CAD build for the part. Positions are in the model's coordinates, mm. A direction names the side the tool comes from. Coordinates: 2 decimals unless noted, no trailing zeros. Loops run counter-clockwise (first coordinate to the right, second up) from the corner with the lowest first, then second, coordinate; pieces in that order, holes last. Notation, with made-up numbers: (56.25, -17) -> (72.25, -17) arc R26 ccw to (72.25, 8) -> close; hole circle Ø4 at (29, 51.5). An arc over 180 degrees is marked (long way). Write each question's results on one line, items separated by ' | '.
```python
from build123d import *

# Parameters (mm, degrees)
F0_R     = 2.75
F0_R_2   = 1.65
F0_W     = 33
F0_H     = 15.5
F0_R_3   = 2.5
F1_DEPTH = 6
F2_R     = 5
F3_DEPTH = 2
F4_DEPTH = 25


with BuildPart() as f1:
    # F0 (on Top) → F1 (new body, symmetric)
    with BuildSketch(Plane.XY):
        Polygon((4, 14.5), (-4, 14.5), (-4, 10.123076), (-4, 5.690599), (0, 3.381198), (4, 5.690599), (4, 10.309401), align=None)
        with Locations((0, 8)):
            Circle(F0_R, mode=Mode.SUBTRACT)
        Polygon((-4, 14.5), (-16.5, 14.5), (-16.5, 1), (16.5, 1), (16.5, 14.5), (4, 14.5), (4, 10.309401), (4, 5.690599), (0, 3.381198), (-4, 5.690599), (-4, 10.123076), align=None)
        with Locations((-10.15, 8)):
            Circle(F0_R_2, mode=Mode.SUBTRACT)
        with Locations((10.15, 8)):
            Circle(F0_R_2, mode=Mode.SUBTRACT)
        with Locations((0, -6.75)):
            Rectangle(F0_W, F0_H)
        with Locations((-10.379309, -9.5)):
            Circle(F0_R_3, mode=Mode.SUBTRACT)
        with Locations((9.157613, -9.5)):
            Circle(F0_R_3, mode=Mode.SUBTRACT)
    extrude(amount=F1_DEPTH, both=True)

    # F2
    f2_edges = [f1.edges().sort_by_distance(p)[0] for p in [
        (16.5, 14.5, 0),
        (-16.5, 14.5, 0),
    ]]
    fillet(f2_edges, radius=F2_R)

    # F0 (on Top) → F3 (cut, symmetric)
    with BuildSketch(Plane.XY):
        Polygon((4, 14.5), (-4, 14.5), (-4, 10.123076), (-4, 5.690599), (0, 3.381198), (4, 5.690599), (4, 10.309401), align=None)
        with Locations((0, 8)):
            Circle(F0_R, mode=Mode.SUBTRACT)
    extrude(amount=F3_DEPTH, both=True, mode=Mode.SUBTRACT)

    # F0 (on Top) → F4 (cut)
    with BuildSketch(Plane.XY):
        with Locations((0, -6.75)):
            Rectangle(F0_W, F0_H)
        with Locations((-10.379309, -9.5)):
            Circle(F0_R_3, mode=Mode.SUBTRACT)
        with Locations((9.157613, -9.5)):
            Circle(F0_R_3, mode=Mode.SUBTRACT)
    extrude(amount=F4_DEPTH, mode=Mode.SUBTRACT)


solid = f1.part
```
Q1. Which spindle directions (+Z, -Z, +X, -X, +Y, -Y) get a long thin tool onto all of the face, cutting with end or side? Do faces 1 (the cylindrical face through (-0.596, 5.315, -4.028)), 2 (the flat face through (0, 11, -2)), 3 (the flat face through (0, -7, 0)). Say none if no direction does.
Results are:
face 1: +Z, -Z | face 2: +Y | face 3: +Z, +X, -X, -Y
Q2. Cut at C-C on z = -0.5. Write the cut outline in (x, y), and give its area (3 significant figures).
Results are:
outline: (-16.5, -14.5) -> (16.5, -14.5) -> (16.5, 9.5) arc R5 ccw to (11.5, 14.5) -> (4, 14.5) -> (4, 5.69) -> (0, 3.38) -> (-4, 5.69) -> (-4, 14.5) -> (-11.5, 14.5) arc R5 ccw to (-16.5, 9.5) -> close; hole circle Ø5 at (-10.38, -9.5); hole circle Ø3.3 at (-10.15, 8); hole circle Ø5 at (9.16, -9.5); hole circle Ø3.3 at (10.15, 8) | area: 810 mm^2
Q3. Pull direction Z, two halves, no side cores. Call faces 4 (the flat face through (0, 5, 6)), 5 (the cylindrical face through (-15.07, 13, -0.08)), 6 (the flat face through (-4, 10, 0)): +Z half, -Z half, draft (parallel to the pull), parting line (faces both ways), or undercut.
Results are:
face 4: +Z half | face 5: draft | face 6: undercut
Q4. Drop flat-ended pins along their axis: pin 1 (5 mm diameter, centred on x = 0, y = 8, fed in from +Z); pin 2 (4.5 mm diameter, centred on x = 3, y = -10, fed in from +Z); pin 3 (1.8 mm diameter, centred on x = 5.5, z = 3.5, fed in from -Y). Give the stop position or say it passes through.
Results are:
pin 1: through | pin 2: z = 0 | pin 3: y = 1
Q5. Cut at A-A on z = -4.5. Write the cut outline in (x, y).
Results are:
outline: (-16.5, -14.5) -> (16.5, -14.5) -> (16.5, 9.5) arc R5 ccw to (11.5, 14.5) -> (-11.5, 14.5) arc R5 ccw to (-16.5, 9.5) -> close; hole circle Ø5 at (-10.38, -9.5); hole circle Ø3.3 at (-10.15, 8); hole circle Ø5.5 at (0, 8); hole circle Ø5 at (9.16, -9.5); hole circle Ø3.3 at (10.15, 8)
Q6. Cut at D-D on y = 8. Write the cut outline in (x, z), and give its area (3 significant figures).
Results are:
outline: (-16.5, -6) -> (-11.8, -6) -> (-11.8, 6) -> (-16.5, 6) -> close; (-8.5, -6) -> (-2.75, -6) -> (-2.75, -2) -> (-4, -2) -> (-4, 2) -> (-2.75, 2) -> (-2.75, 6) -> (-8.5, 6) -> close; (2.75, -6) -> (8.5, -6) -> (8.5, 6) -> (2.75, 6) -> (2.75, 2) -> (4, 2) -> (4, -2) -> (2.75, -2) -> close; (11.8, -6) -> (16.5, -6) -> (16.5, 6) -> (11.8, 6) -> close | area: 241 mm^2
Q7. Wall check: L1, parallel to X at y = 6, z = -1.5; L2, parallel to Y at x = 9.5, z = -4.5; L3, parallel to Z at x = 0.5, y = 10.75. Give the ranges that are in metal, low to high. Write a range as from..to.
Results are:
L1: -16.5..-4, 4..16.5 | L2: -14.5..-11.98, -7.02..6.48, 9.52..14.5 | L3: -6..-2, 2..6
Q8. Cut at B-B on x = 11. Write the cut outline in (y, z).
Results are:
outline: (-14.5, -6) -> (-11.19, -6) -> (-11.19, 0) -> (-14.5, 0) -> close; (-7.81, -6) -> (6.59, -6) -> (6.59, 6) -> (1, 6) -> (1, 0) -> (-7.81, 0) -> close; (9.41, -6) -> (14.5, -6) -> (14.5, 6) -> (9.41, 6) -> close
